Geometry: final body of the model. Coordinates: model frame, mm. Face numbers are marked on the shaded views. Round coordinates to 2 decimals unless told otherwise and drop trailing zeros. Write each loop counter-clockwise with the first axis right and the second up, starting at its lowest first coordinate (ties: lowest second). Pieces come first, ordered by that corner, then holes. Notation, with made-up numbers: M 49.5,-19 L 89.5,-19 A23 cw 89.5,14 Z; hole C 87,69.25 d5. An arc over 180 degrees is marked long. Answer as CSV lines item,"result". Start each with the question number.
Q1. Ray query, probe 1 along X at (y, z) = (-85, 28); probe 2 along Y at (x, z) = (259, 39); probe 3 along Z at (x, y) = (512.6, -127). Return the intervals inside material, ascending.
Q2. Section query C-C on x = -420.5. Output: boundary loops of the cut face in (y, z), and give its area (3 significant figures).
Q3. First-contact query: pin 1 (4 mm diameter, centred on y = -127, z = 24.892, fed in from -X); pin 2 (1 mm diameter, centred on x = -53, y = -108.5, fed in from +Z). Flat tips, straight axial feed; report the tip coordinate or a pass-through.
Q4. Section query B-B on y = -14.5. Output: boundary loops of the cut face in (x, z).
Q5. Section query A-A on z = 42. Output: boundary loops of the cut face in (x, y).
Q6. Mould query, pull axis X, two halves, no side actions, for the marked faces 1, 2 and 3. Classes: pulls with the +X half, pulls with the -X half, needs draft (parallel to the pull), parting line crosses it, or undercut.
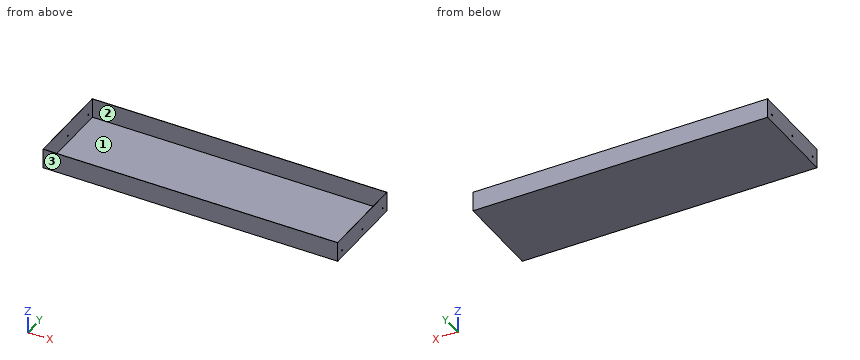
```python
from build123d import *

# Parameters (mm, degrees)
F0_W     = 1026.16
F0_H     = 308.356
F1_DEPTH = 68.58
F2_T     = -0.762
F4_D     = 5.2197


with BuildPart() as f1:
    # F0 (on Top) → F1 (new body)
    with BuildSketch(Plane.XY):
        Rectangle(F0_W, F0_H)
    extrude(amount=F1_DEPTH)

    # F2
    f2_openings = [f1.faces().sort_by_distance(p)[0] for p in [
        (0, 0, 68.58),
    ]]
    offset(amount=F2_T, openings=f2_openings)

    # F4 (through all)
    with Locations(Plane(origin=(-513.08, 0, 0), x_dir=(0, -1, 0), z_dir=(-1, 0, 0))):
        with Locations((-127, 24.892), (0, 24.892), (127, 24.892)):
            Hole(F4_D / 2)


solid = f1.part
```
Entries:
1,probe 1,"x = -513.08 to -512.32, 512.32 to 513.08"
1,probe 2,"y = -154.18 to -153.42, 153.42 to 154.18"
1,probe 3,"z = 0 to 22.28, 27.5 to 68.58"
2,outline,"M -154.18,0 L 154.18,0 L 154.18,68.58 L 153.42,68.58 L 153.42,0.76 L -153.42,0.76 L -153.42,68.58 L -154.18,68.58 Z"
2,area,"338 mm^2"
3,pin 1,"passes through"
3,pin 2,"stops at z = 0.76"
4,outline,"M -513.08,0 L 513.08,0 L 513.08,68.58 L 512.32,68.58 L 512.32,0.76 L -512.32,0.76 L -512.32,68.58 L -513.08,68.58 Z"
5,outline,"M -513.08,-154.18 L 513.08,-154.18 L 513.08,154.18 L -513.08,154.18 Z; hole M -512.32,-153.42 L 512.32,-153.42 L 512.32,153.42 L -512.32,153.42 Z"
6,face 1,"undercut"
6,face 2,"undercut"
6,face 3,"needs draft"
